Design review of the part built by this model. Coordinates are the model's own, in mm. A direction names the side the tool comes from. Round coordinates to 2 decimals unless told otherwise and drop trailing zeros. Loops run counter-clockwise (first coordinate to the right, second up) from the corner with the lowest first, then second, coordinate; pieces in that order, holes last. Notation, with made-up numbers: (72, -23.5) -> (86, -23.5) arc R14 ccw to (86, -6.5) -> close; hole circle Ø8 at (16, 24). An arc over 180 degrees is marked (long way). Write each question's results on one line, items separated by ' | '. Start each with the question number.
Autodesk Inventor part; units mm, degrees
ref_plane "YZ Plane" through (0, 0, 0) normal (1, 0, 0) x (0, 1, 0)
ref_plane "XZ Plane" through (0, 0, 0) normal (0, 1, 0) x (-1, 0, 0)
ref_plane "XY Plane" through (0, 0, 0) normal (0, 0, 1) x (1, 0, 0)
sketch "Sketch1" plane through (0, 0, 0) normal (0, 0, 1) x (1, 0, 0)
  point P0 (0, 0)
sketch "Sketch2" plane through (0, 0, 0) normal (0, 0, 1) x (1, 0, 0)
  line L0 (0, 0) -> (75, 0)
  line L1 (75, 0) -> (75, 50)
  line L2 (75, 50) -> (0, 50)
  line L3 (0, 50) -> (0, 0)
  dimension "d0" = 75
  dimension "d1" = 50
extrude "Extrusion1" add sketch "Sketch2" along normal blind 15
sketch "Sketch3" plane through (0, 0, 0) normal (0, 0, -1) x (-1, 0, 0)
  line L0 (0, 50) -> (0, 0)
  circle A0 centre (0, 25) radius 25
extrude "Extrusion2" add sketch "Sketch3" against normal blind 40
sketch "Sketch4" plane through (0, 25, 40) normal (0, 0, 1) x (1, 0, 0)
  circle A0 centre (0, 0) radius 25
  circle A1 centre (0, 0) radius 15
  point P0 (0, -25)
  dimension "d6" = 30
extrude "Extrusion3" cut sketch "Sketch4" against normal through all contours A1
hole "Hole1" at (45, 25, 15) direction (0, 0, -1) diameter 20 end through all
sketch "Sketch5" plane through (75, 0, 0) normal (1, 0, 0) x (0, 0, -1)
  line L0 (0, 15) -> (-15, 15)
  line L1 (-15, 15) -> (0, 15)
  line L2 (0, 15) -> (0, 35)
  line L3 (0, 35) -> (-15, 35)
  line L4 (-15, 35) -> (-15, 15)
  dimension "d19" = 20
  dimension "d20" = 15
extrude "Extrusion4" cut sketch "Sketch5" against normal up to next
properties part number "Locator"
1) The part is to be moulded in two halves that separate along X. For faces 1 (the face through (-23.09, 15.42, 24.16)), 2 (the face through (-3.252, 10.357, 20.28)), 3 (the face through (60, 15, 7)), 4 (the face through (75, 7, 7)), say which applies: +X half, -X half, draft (parallel to the pull), parting line (faces both ways), or undercut.
2) Insertion check: pin 1 (4 mm diameter, centred on y = 38.5, z = 28.5, fed in from -X); pin 2 (24 mm diameter, centred on x = 0, y = 25, fed in from -Z); pin 3 (5 mm diameter, centred on y = 17.5, z = 33.5, fed in from +X); pin 4 (1 mm diameter, centred on x = 21.5, z = 28, fed in from +Y). Each pin has a flat end and moves straight along its axis. Give the tip position at first contact, or say it passes through.
3) To check wall thickness, follow line 1 (Y direction, x = 0, z = 19); line 2 (Z direction, x = 12, y = 48.5); line 3 (Y direction, x = 53.5, z = 8). State the ranges of each line that lie inside material, in increasing order. Write a range as from..to.
4) Take a section at A-A (x = 62.5). Write out the cut boundary in (y, z).
5) For faces 5 (the face through (24, 25, 0)), 6 (the face through (60, 35, 7)), list the 3-axis set-ups (+Z, -Z, +X, -X, +Y, -Y) from which the entire face can be reached by the end or side of a thin tool; tool diameter is ignored.
6) Take a section at C-C (z = 4). Write out the cut boundary in (x, y).
7) Take a section at B-B (y = 25). Write out the cut boundary in (x, z), plus the area to 3 significant figures.
Geometry check:
1) face 1: parting line | face 2: undercut | face 3: draft | face 4: +X half
2) pin 1: stops at x = -22.2 | pin 2: passes through | pin 3: stops at x = 24.49 | pin 4: stops at y = 38.56
3) line 1: y = 0..10, 40..50 | line 2: z = 0..15 | line 3: y = 0..15, 35..50
4) outline: (0, 0) -> (15, 0) -> (15, 15) -> (0, 15) -> close; (35, 0) -> (50, 0) -> (50, 15) -> (35, 15) -> close
5) face 5: -Z, +X, -X, +Y, -Y | face 6: +Z, -Z, +X
6) outline: (0, 0) -> (75, 0) -> (75, 15) -> (45, 15) arc R10 cw to (45, 35) -> (75, 35) -> (75, 50) -> (0, 50) arc R25 ccw to start; hole circle Ø30 at (0, 25)
7) outline: (-25, 0) -> (-15, 0) -> (-15, 40) -> (-25, 40) -> close; (15, 0) -> (35, 0) -> (35, 15) -> (25, 15) -> (25, 40) -> (15, 40) -> close | area: 950 mm^2
